Verification items for the finished model (mm, model axes). Give positions to 0.01 mm unless a question says otherwise; leave off trailing zeros. Loops run counter-clockwise (first coordinate to the right, second up) from the corner with the lowest first, then second, coordinate; pieces in that order, holes last. Notation, with made-up numbers: (-26.75, 18.5) - (-3.75, 18.5) arc R18 ccw to (-3.75, 49.5) - close; hole circle Ø4 at (-7.5, 21.25). An arc over 180 degrees is marked (long way). One line per item, written item: value. Start each with the question number.
1. Gauge pin test, flat ends, axial feed: pin 1 (5 mm diameter, centred on x = 9.5, z = 16.5, fed in from -Y); pin 2 (10 mm diameter, centred on x = 0, z = -26.5, fed in from -Y); pin 3 (10 mm diameter, centred on x = 14, z = 2.5, fed in from -Y). Record the tip position at first contact, or that the pin passes through.
2. Scan lines: L1, parallel to Y at x = -5, z = -31; L2, parallel to Y at x = -5.5, z = -34.5. Record each from-to range of solid material in increasing order. Write a range as [from, to].
3. Sectioned sample at A-A (x = 12). Record the cut outline in (y, z).
4. Sectioned sample at B-B (z = -5.5). Record the cut outline in (x, y), plus the area to 3 significant figures.
from build123d import *

# Parameters (mm, degrees)
F0_W     = 38.1
F0_H     = 88.9
F1_DEPTH = 972.82
F3_DEPTH = 25.4
F5_DEPTH = 25.4


with BuildPart() as f1:
    # F0 (on Front) → F1 (new body)
    with BuildSketch(Plane.XZ):
        Rectangle(F0_W, F0_H)
    extrude(amount=F1_DEPTH)

    # F2 (on Right) → F3 (cut, symmetric)
    with BuildSketch(Plane.YZ):
        Polygon((-972.82, -44.45), (-948.944, 44.45), (-972.82, 44.45), align=None)
    extrude(amount=F3_DEPTH, both=True, mode=Mode.SUBTRACT)

    # F4 (on Right) → F5 (cut, symmetric)
    with BuildSketch(Plane.YZ):
        Polygon((0, -44.45), (0, 44.45), (-23.876, -44.45), align=None)
    extrude(amount=F5_DEPTH, both=True, mode=Mode.SUBTRACT)


solid = f1.part
Results are:
1. pin 1: stops at y = -957.12
1. pin 2: stops at y = -969.34
1. pin 3: stops at y = -961.55
2. L1: y = [-969.21, -20.26]
2. L2: y = [-970.15, -21.2]
3. outline: (-972.82, -44.45) - (-23.88, -44.45) - (0, 44.45) - (-948.94, 44.45) - close
4. outline: (-19.05, -962.36) - (19.05, -962.36) - (19.05, -13.42) - (-19.05, -13.42) - close
4. area: 36,200 mm^2
